```python
from build123d import *

# Parameters (mm, degrees)
BOSS_EXTRUDE1_DEPTH      = 150
BOSS_EXTRUDE1_DEPTH_BACK = 150
SKETCH1_W                = 500
SKETCH1_H                = 300
SKETCH2_W                = 40
SKETCH2_H                = 40
BOSS_EXTRUDE2_DEPTH      = 20
SKETCH3_W                = 20
SKETCH3_H                = 1000
BOSS_EXTRUDE3_DEPTH      = 340
FILLET1_R                = 10
SKETCH4_R                = 40
BOSS_EXTRUDE4_DEPTH      = 150
SKETCH5_R                = 10
BOSS_EXTRUDE5_DEPTH      = 50
FILLET1_OF_MIRROR1_R     = 10
SKETCH7_R                = 150
BOSS_EXTRUDE6_DEPTH      = 300


with BuildPart() as part:
    # Sketch1 → Boss-Extrude1 (new, two sides: drawn at the far end of the back side and taken through both)
    with BuildSketch(Plane.XY.offset(-BOSS_EXTRUDE1_DEPTH_BACK)):
        Rectangle(SKETCH1_W, SKETCH1_H)
    extrude(amount=BOSS_EXTRUDE1_DEPTH + BOSS_EXTRUDE1_DEPTH_BACK)

    # Sketch2 → Boss-Extrude2 (add)
    with BuildSketch(Plane.XY.offset(150)):
        Rectangle(SKETCH2_W, SKETCH2_H)
    boss_extrude2 = extrude(amount=BOSS_EXTRUDE2_DEPTH)

    # Sketch3 → Boss-Extrude3 (add)
    with BuildSketch(Plane.XY.offset(170)):
        Rectangle(SKETCH3_W, SKETCH3_H)
    boss_extrude3 = extrude(amount=BOSS_EXTRUDE3_DEPTH)

    # Fillet1
    fillet1_edges = [part.edges().sort_by_distance(p)[0] for p in [
        (-10, 0, 170),
        (10, 0, 170),
    ]]
    fillet(fillet1_edges, radius=FILLET1_R - 0.0001)  # a hair under: the kernel refuses the full size

    # Sketch4 → Boss-Extrude4 (add)
    with BuildSketch(Plane.ZY.offset(250)):
        with Locations((58.043987529, 0)):
            Circle(SKETCH4_R)
    boss_extrude4 = extrude(amount=BOSS_EXTRUDE4_DEPTH)

    # Sketch5 → Boss-Extrude5 (add)
    with BuildSketch(Plane.ZY.offset(400)):
        with Locations((58.043987529, 0)):
            Circle(SKETCH5_R)
    boss_extrude5 = extrude(amount=BOSS_EXTRUDE5_DEPTH)

    # Mirror1: Boss-Extrude2, Boss-Extrude3, Boss-Extrude4, Boss-Extrude5 across plane
    add(boss_extrude2.mirror(Plane.XY))
    add(boss_extrude3.mirror(Plane.XY))
    add(boss_extrude4.mirror(Plane.XY))
    add(boss_extrude5.mirror(Plane.XY))

    # Fillet1 of Mirror1
    fillet1_of_mirror1_edges = [part.edges().sort_by_distance(p)[0] for p in [
        (-10, 0, -170),
        (10, 0, -170),
    ]]
    fillet(fillet1_of_mirror1_edges, radius=FILLET1_OF_MIRROR1_R - 0.0001)  # a hair under: the kernel refuses the full size

    # Sketch7 → Boss-Extrude6 (add)
    with BuildSketch(Plane(origin=(250, 0, 0), x_dir=(0, 0, -1), z_dir=(1, 0, 0))):
        Circle(SKETCH7_R)
    extrude(amount=BOSS_EXTRUDE6_DEPTH)


solid = part.part
```
Work out the finished part from the listing and answer in its coordinate system (mm). A direction names the side the tool comes from. Coordinates: 2 decimals unless noted, no trailing zeros. Write each loop counter-clockwise with the first axis right and the second up, starting at its lowest first coordinate (ties: lowest second). Pieces come first, ordered by that corner, then holes.
Q1. Determine the mould class of faces 1 (the face through (397.9, 148.724, 19.527)), 2 (the face through (250, 114, -120)), 3 (the face through (0, -20, 161)) for opening direction Z: released by +Z, released by -Z, zero draft, split by the parting line, or undercut.
Q2. Which of the six approach directions +Z, -Z, +X, -X, +Y, -Y give full straight-line access (tool end or side, diameter ignored) to faces 4 (the face through (250, 119, 119)), 5 (the face through (250, -120, 114)), 6 (the face through (-323.95, -39.05, 49.37)), 7 (the face through (250, -120, -114)), 8 (the face through (550, 2, 2))?
Q3. Find the intervals of material crossed by line 1 (X direction, y = 93, z = 76); line 2 (X direction, y = -15, z = -367); line 3 (Z direction, x = 105.5, y = -45), in increasing order.
Q4. Each of these flat-tipped pins is pushed along its axis until it touches: pin 1 Ø22 at (y, z) = (3, -159) entering from -X; pin 2 Ø2 at (x, y) = (13, -70) entering from -Z; pin 3 Ø9 at (x, z) = (-9, -161.5) entering from -Y. Where does it stop, or does it pass through?
Q5. A cutting plane is placed at A-A, the plane y = -200. Give the vertices of the cut face in (x, z).
Q6. A cutting plane is placed at B-B, the plane x = -321. Give the vertices of the cut face in (y, z).
Q7. A cutting plane is placed at D-D, the plane x = 438. Give the vertices of the cut face in (y, z), then the cut area to 3 significant figures.
Q8. A cutting plane is placed at C-C, the plane y = -93.5. Give the vertices of the cut face in (x, z), then the cut area to 3 significant figures.
Findings below:
1. face 1: split by the parting line
1. face 2: zero draft
1. face 3: undercut
2. face 4: +Z, +X, +Y
2. face 5: +Z, +X, -Y
2. face 6: -X
2. face 7: -Z, +X, -Y
2. face 8: +Z, -Z, +X, +Y, -Y
3. line 1: x = -250 to 550
3. line 2: x = -10 to 10
3. line 3: z = -150 to 150
4. pin 1: stops at x = -250
4. pin 2: stops at z = -150
4. pin 3: stops at y = -20
5. outline: (-10, -510) - (10, -510) - (10, -170) - (-10, -170) - close; (-10, 170) - (10, 170) - (10, 510) - (-10, 510) - close
6. outline: circle Ø80 at (0, -58.04); circle Ø80 at (0, 58.04)
7. outline: circle Ø300 at (0, 0)
7. area: 70,700 mm2
8. outline: (-250, -150) - (250, -150) - (250, -117.29) - (550, -117.29) - (550, 117.29) - (250, 117.29) - (250, 150) - (-250, 150) - close; (-10, -510) - (10, -510) - (10, -170) - (-10, -170) - close; (-10, 170) - (10, 170) - (10, 510) - (-10, 510) - close
8. area: 234,000 mm2
